Here's how the part is built. I have some questions about the finished solid (model axes, mm). Round coordinates to 2 decimals unless told otherwise and drop trailing zeros. Loops run counter-clockwise (first coordinate to the right, second up) from the corner with the lowest first, then second, coordinate; pieces in that order, holes last. Notation, with made-up numbers: (8, 47) - (39, 47) arc R17 cw to (39, 72) - close; hole circle Ø9 at (13.5, 81). An arc over 180 degrees is marked (long way). Return JSON: item names as keys, results as strings. Group by question number.
```python
from build123d import *

# Parameters (mm, degrees)
F0_R     = 24.003
F0_R_2   = 3.054646
F1_DEPTH = 2.54


with BuildPart() as f1:
    # F0 (on Top) → F1 (new body)
    with BuildSketch(Plane.XY):
        Circle(F0_R)
        with BuildLine():
            ThreePointArc((1.17752, -20.066034), (0, -20.100554), (-1.17752, -20.066034))
            Line((-1.17752, -20.066034), (-10.217665, -11.025888))
            Line((-10.217665, -11.025888), (-8.177547, -10.621777))
            ThreePointArc((-8.177547, -10.621777), (0, -13.405015), (8.177547, -10.621777))
            Line((8.177547, -10.621777), (10.217665, -11.025888))
            Line((10.217665, -11.025888), (1.17752, -20.066034))
        make_face(mode=Mode.SUBTRACT)
        with BuildLine():
            ThreePointArc((-0.5715, -22.852855), (-16.164461, -16.164461), (-22.852855, -0.5715))
            Line((-22.852855, -0.5715), (-21.176763, -1.683237))
            ThreePointArc((-21.176763, -1.683237), (-15.021461, -15.021461), (-1.683237, -21.176763))
            Line((-1.683237, -21.176763), (-0.5715, -22.852855))
        make_face(mode=Mode.SUBTRACT)
        with BuildLine():
            Line((-19.87815, -2.98185), (-2.98185, -19.87815))
            ThreePointArc((-2.98185, -19.87815), (-14.213238, -14.213238), (-19.87815, -2.98185))
        make_face(mode=Mode.SUBTRACT)
        with BuildLine():
            ThreePointArc((-10.621777, -6.12657), (-12.262015, 0), (-10.621777, 6.12657))
            Line((-10.621777, 6.12657), (-10.621777, -6.12657))
        make_face(mode=Mode.SUBTRACT)
        with BuildLine():
            Line((-0.5715, -9.478777), (-7.778804, -9.478777))
            ThreePointArc((-7.778804, -9.478777), (-8.670554, -8.670554), (-9.478777, -7.778804))
            Line((-9.478777, -7.778804), (-9.478777, -0.5715))
            Line((-9.478777, -0.5715), (-8.907277, -0.5715))
            Line((-8.907277, -0.5715), (-7.645644, -1.833133))
            Line((-7.645644, -1.833133), (-1.833133, -7.645644))
            Line((-1.833133, -7.645644), (-0.808231, -8.670546))
            Line((-0.808231, -8.670546), (-0.5715, -8.907277))
            Line((-0.5715, -8.907277), (-0.5715, -9.478777))
        make_face(mode=Mode.SUBTRACT)
        with BuildLine():
            Line((-0.5715, -7.290831), (-7.290831, -0.5715))
            Line((-7.290831, -0.5715), (-4.15856, -0.5715))
            ThreePointArc((-4.15856, -0.5715), (-2.968184, -2.968184), (-0.5715, -4.15856))
            Line((-0.5715, -4.15856), (-0.5715, -7.290831))
        make_face(mode=Mode.SUBTRACT)
        with BuildLine():
            ThreePointArc((6.12657, -10.621777), (0, -12.262015), (-6.12657, -10.621777))
            Line((-6.12657, -10.621777), (6.12657, -10.621777))
        make_face(mode=Mode.SUBTRACT)
        with BuildLine():
            ThreePointArc((22.852855, -0.5715), (16.164461, -16.164461), (0.5715, -22.852855))
            Line((0.5715, -22.852855), (1.683237, -21.176763))
            ThreePointArc((1.683237, -21.176763), (15.021461, -15.021461), (21.176763, -1.683237))
            Line((21.176763, -1.683237), (22.852855, -0.5715))
        make_face(mode=Mode.SUBTRACT)
        with BuildLine():
            ThreePointArc((19.87815, -2.98185), (14.213238, -14.213238), (2.98185, -19.87815))
            Line((2.98185, -19.87815), (19.87815, -2.98185))
        make_face(mode=Mode.SUBTRACT)
        with BuildLine():
            Line((0.5715, -9.478777), (0.5715, -8.902199))
            Line((0.5715, -8.902199), (0.804649, -8.666979))
            Line((0.804649, -8.666979), (8.828836, -0.5715))
            Line((8.828836, -0.5715), (9.478777, -0.5715))
            Line((9.478777, -0.5715), (9.478777, -7.778804))
            ThreePointArc((9.478777, -7.778804), (8.670554, -8.670554), (7.778804, -9.478777))
            Line((7.778804, -9.478777), (0.5715, -9.478777))
        make_face(mode=Mode.SUBTRACT)
        with BuildLine():
            Line((7.219491, -0.5715), (0.5715, -7.278557))
            Line((0.5715, -7.278557), (0.5715, -4.15856))
            ThreePointArc((0.5715, -4.15856), (2.968184, -2.968184), (4.15856, -0.5715))
            Line((4.15856, -0.5715), (7.219491, -0.5715))
        make_face(mode=Mode.SUBTRACT)
        with BuildLine():
            ThreePointArc((20.066034, 1.17752), (20.100554, 0), (20.066034, -1.17752))
            Line((20.066034, -1.17752), (11.025888, -10.217665))
            Line((11.025888, -10.217665), (10.621777, -8.177547))
            ThreePointArc((10.621777, -8.177547), (13.405015, 0), (10.621777, 8.177547))
            Line((10.621777, 8.177547), (11.025888, 10.217665))
            Line((11.025888, 10.217665), (20.066034, 1.17752))
        make_face(mode=Mode.SUBTRACT)
        with BuildLine():
            ThreePointArc((-20.066034, -1.17752), (-20.100554, 0), (-20.066034, 1.17752))
            Line((-20.066034, 1.17752), (-11.025888, 10.217665))
            Line((-11.025888, 10.217665), (-10.621777, 8.177547))
            ThreePointArc((-10.621777, 8.177547), (-13.405015, 0), (-10.621777, -8.177547))
            Line((-10.621777, -8.177547), (-11.025888, -10.217665))
            Line((-11.025888, -10.217665), (-20.066034, -1.17752))
        make_face(mode=Mode.SUBTRACT)
        with BuildLine():
            Line((-7.294226, 0.568104), (-0.5715, 7.290831))
            Line((-0.5715, 7.290831), (-0.5715, 4.15856))
            ThreePointArc((-0.5715, 4.15856), (-2.971748, 2.964616), (-4.159921, 0.561506))
            Line((-4.159921, 0.561506), (-7.294226, 0.568104))
        make_face(mode=Mode.SUBTRACT)
        with BuildLine():
            ThreePointArc((-9.478777, 7.778804), (-8.670554, 8.670554), (-7.778804, 9.478777))
            Line((-7.778804, 9.478777), (-0.5715, 9.478777))
            Line((-0.5715, 9.478777), (-0.5715, 8.907277))
            Line((-0.5715, 8.907277), (-1.833133, 7.645644))
            Line((-1.833133, 7.645644), (-7.645644, 1.833133))
            Line((-7.645644, 1.833133), (-8.907277, 0.5715))
            Line((-8.907277, 0.5715), (-9.478777, 0.5715))
            Line((-9.478777, 0.5715), (-9.478777, 7.778804))
        make_face(mode=Mode.SUBTRACT)
        with BuildLine():
            Line((-2.98185, 19.87815), (-19.87815, 2.98185))
            ThreePointArc((-19.87815, 2.98185), (-14.213238, 14.213238), (-2.98185, 19.87815))
        make_face(mode=Mode.SUBTRACT)
        with BuildLine():
            ThreePointArc((-1.683237, 21.176763), (-15.021461, 15.021461), (-21.176763, 1.683237))
            Line((-21.176763, 1.683237), (-22.852855, 0.5715))
            ThreePointArc((-22.852855, 0.5715), (-16.164461, 16.164461), (-0.5715, 22.852855))
            Line((-0.5715, 22.852855), (-1.683237, 21.176763))
        make_face(mode=Mode.SUBTRACT)
        with BuildLine():
            Line((6.12657, 10.621777), (-6.12657, 10.621777))
            ThreePointArc((-6.12657, 10.621777), (0, 12.262015), (6.12657, 10.621777))
        make_face(mode=Mode.SUBTRACT)
        with BuildLine():
            ThreePointArc((-1.17752, 20.066034), (0, 20.100554), (1.17752, 20.066034))
            Line((1.17752, 20.066034), (10.217665, 11.025888))
            Line((10.217665, 11.025888), (8.177547, 10.621777))
            ThreePointArc((8.177547, 10.621777), (0, 13.405015), (-8.177547, 10.621777))
            Line((-8.177547, 10.621777), (-10.217665, 11.025888))
            Line((-10.217665, 11.025888), (-1.17752, 20.066034))
        make_face(mode=Mode.SUBTRACT)
        Circle(F0_R_2, mode=Mode.SUBTRACT)
        with BuildLine():
            Line((0.5715, 7.290831), (7.325001, 0.53733))
            Line((7.325001, 0.53733), (4.162248, 0.543987))
            ThreePointArc((4.162248, 0.543987), (2.977982, 2.958354), (0.5715, 4.15856))
            Line((0.5715, 4.15856), (0.5715, 7.290831))
        make_face(mode=Mode.SUBTRACT)
        with BuildLine():
            ThreePointArc((7.778804, 9.478777), (8.670554, 8.670554), (9.478777, 7.778804))
            Line((9.478777, 7.778804), (9.478777, 0.5715))
            Line((9.478777, 0.5715), (8.907277, 0.5715))
            Line((8.907277, 0.5715), (7.645644, 1.833133))
            Line((7.645644, 1.833133), (1.833133, 7.645644))
            Line((1.833133, 7.645644), (0.5715, 8.907277))
            Line((0.5715, 8.907277), (0.5715, 9.478777))
            Line((0.5715, 9.478777), (7.778804, 9.478777))
        make_face(mode=Mode.SUBTRACT)
        with BuildLine():
            ThreePointArc((10.621777, 6.12657), (12.262015, 0), (10.621777, -6.12657))
            Line((10.621777, -6.12657), (10.621777, 6.12657))
        make_face(mode=Mode.SUBTRACT)
        with BuildLine():
            Line((19.87815, 2.98185), (2.98185, 19.87815))
            ThreePointArc((2.98185, 19.87815), (14.213238, 14.213238), (19.87815, 2.98185))
        make_face(mode=Mode.SUBTRACT)
        with BuildLine():
            ThreePointArc((0.5715, 22.852855), (16.164461, 16.164461), (22.852855, 0.5715))
            Line((22.852855, 0.5715), (21.176763, 1.683237))
            ThreePointArc((21.176763, 1.683237), (15.021461, 15.021461), (1.683237, 21.176763))
            Line((1.683237, 21.176763), (0.5715, 22.852855))
        make_face(mode=Mode.SUBTRACT)
    extrude(amount=F1_DEPTH)


solid = f1.part
```
Q1. Imagine slicing it at A-A, the plane x = 0. List the corners of the cut face in (y, z) for me, and give its area (3 significant figures).
Q2. Imagine slicing it at C-C, the plane z = 0.95. Give the number of separate pieces and of enclosed holes in the cut face, and give its area (3 significant figures).
Q3. Please list where these lines run through material, in increasing order: line 1 (Y direction, x = 16, z = 1.2); line 2 (X direction, y = 17, z = 1.9); line 3 (Y direction, x = 18, z = 1.6).
Q4. Imagine slicing it at B-B, the plane y = 14.5. List the corners of the cut face in (x, z) for me, and give its area (3 significant figures).
Q5. Will these pins go through, and if not, where does the flat tip stop? pin 1 Ø0.8 at (x, z) = (-1.5, 1) entering from -Y; pin 2 Ø1.3 at (y, z) = (2, 1.5) entering from -X (3 decimals); pin 3 Ø0.5 at (y, z) = (9, 1) entering from -X.
Output values:
{
 "1": {"outline": "(-24, 0) - (-20.1, 0) - (-20.1, 2.54) - (-24, 2.54) - close; (-13.41, 0) - (-12.26, 0) - (-12.26, 2.54) - (-13.41, 2.54) - close; (-10.62, 0) - (-3.05, 0) - (-3.05, 2.54) - (-10.62, 2.54) - close; (3.05, 0) - (10.62, 0) - (10.62, 2.54) - (3.05, 2.54) - close; (12.26, 0) - (13.41, 0) - (13.41, 2.54) - (12.26, 2.54) - close; (20.1, 0) - (24, 0) - (24, 2.54) - (20.1, 2.54) - close", "area": "64.1 mm^2"},
 "2": {"separate pieces": "1", "enclosed holes": "25", "area": "717 mm^2"},
 "3": {"line 1": "y = -17.89 to -16.33, -13.97 to -12.17, -6.86 to -5.24, 5.24 to 6.86, 12.17 to 13.97, 16.33 to 17.89", "line 2": "x = -16.95 to -15.28, -12.74 to -10.73, -5.86 to -4.24, 4.24 to 5.86, 10.73 to 12.74, 15.28 to 16.95", "line 3": "y = -15.88 to -14.09, -11.28 to -8.95, -4.86 to -3.24, 3.24 to 4.86, 8.95 to 11.28, 14.09 to 15.88"},
 "4": {"outline": "(-19.13, 0) - (-17.67, 0) - (-17.67, 2.54) - (-19.13, 2.54) - close; (-15.53, 0) - (-13.92, 0) - (-13.92, 2.54) - (-15.53, 2.54) - close; (-8.36, 0) - (-6.74, 0) - (-6.74, 2.54) - (-8.36, 2.54) - close; (6.74, 0) - (8.36, 0) - (8.36, 2.54) - (6.74, 2.54) - close; (13.92, 0) - (15.53, 0) - (15.53, 2.54) - (13.92, 2.54) - close; (17.67, 0) - (19.13, 0) - (19.13, 2.54) - (17.67, 2.54) - close", "area": "23.8 mm^2"},
 "5": {"pin 1": "stops at y = -23.98", "pin 2": "stops at x = -23.965", "pin 3": "stops at x = -22.35"}
}
